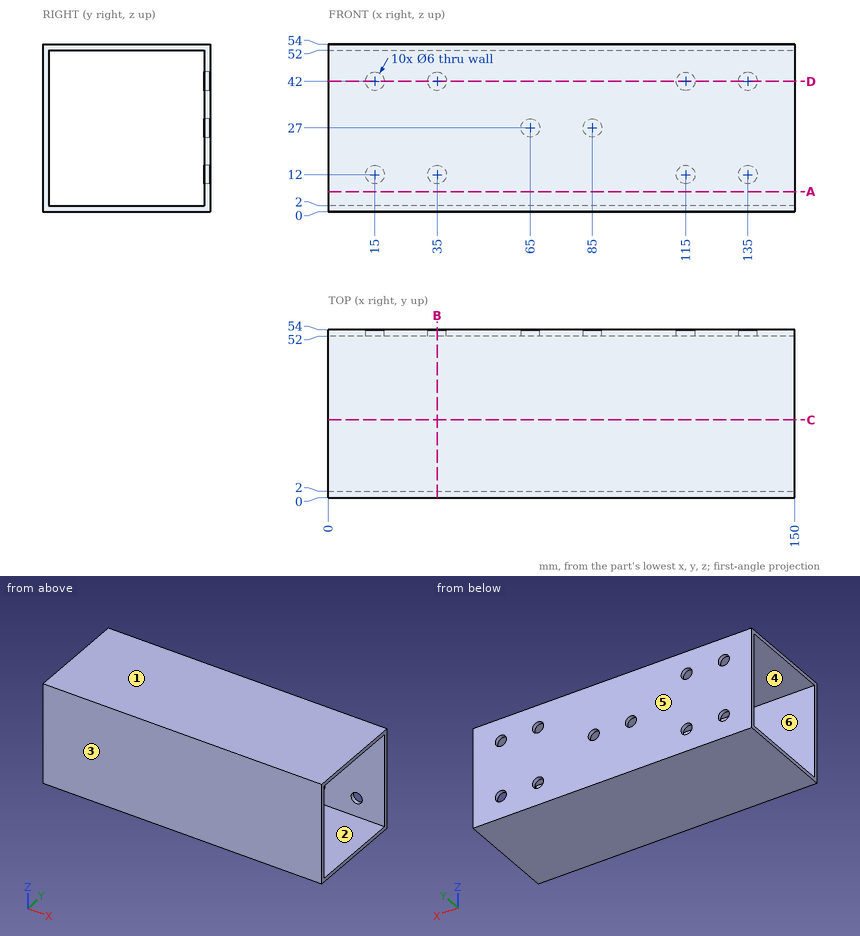
Answer from the drawing. Dimensions are ordinates in mm from the lowest x, y and z of the part. A direction names the side the tool comes from. Round coordinates to 2 decimals unless told otherwise and drop trailing zeros. Loops run counter-clockwise (first coordinate to the right, second up) from the corner with the lowest first, then second, coordinate; pieces in that order, holes last.
(1) Each of these flat-tipped pins is pushed along its axis until it touches: P1, Ø5, axis at y = 48, z = 31, coming from the -X side; P2, Ø3.5, axis at x = 85, z = 27, coming from the +Y side. Where does it stop, or does it pass through?
Computed values:
P1: passes through
P2: stops at y = 2
(2) The part is cut by section A-A, the plane z = 6.5. Give the vertices of the cut face in (x, y), and give its area (3 significant figures).
Computed values:
outline: (0, 0) - (150, 0) - (150, 2) - (0, 2) - close; (0, 52) - (150, 52) - (150, 54) - (0, 54) - close
area: 600 mm2
(3) The mould has two halves that part along Y. Classify the marked faces 3, 4, 5 and 6: pulls with the +Y half, pulls with the -Y half, needs draft (parallel to the pull), parting line crosses it, or undercut.
Computed values:
face 3: pulls with the -Y half
face 4: undercut
face 5: pulls with the +Y half
face 6: undercut
(4) The part is cut by section D-D, the plane z = 42. Give the vertices of the cut face in (x, y).
Computed values:
outline: (0, 0) - (150, 0) - (150, 2) - (0, 2) - close; (0, 52) - (12, 52) - (12, 54) - (0, 54) - close; (18, 52) - (32, 52) - (32, 54) - (18, 54) - close; (38, 52) - (112, 52) - (112, 54) - (38, 54) - close; (118, 52) - (132, 52) - (132, 54) - (118, 54) - close; (138, 52) - (150, 52) - (150, 54) - (138, 54) - close
(5) The part is cut by section B-B, the plane x = 35. Give the vertices of the cut face in (y, z), and give its area (3 significant figures).
Computed values:
outline: (0, 0) - (54, 0) - (54, 9) - (52, 9) - (52, 2) - (2, 2) - (2, 52) - (52, 52) - (52, 45) - (54, 45) - (54, 54) - (0, 54) - close; (52, 15) - (54, 15) - (54, 39) - (52, 39) - close
area: 392 mm2
(6) Find the intervals of material crossed by L1, parallel to Z at x = 115, y = 52.75; L2, parallel to Y at x = 96, z = 30, in increasing order.
Computed values:
L1: z = 0 to 9, 15 to 39, 45 to 54
L2: y = 0 to 2, 52 to 54
(7) For the marked faces 1 and 2, determine the directions among +Z, -Z, +X, -X, +Y, -Y from which every point of the face is accessible in a straight line to the end or side of a thin tool.
Computed values:
face 1: +Z, +X, -X, +Y, -Y
face 2: +X, -X
